Input: dimensioned drawing with shaded views. Units: mm. Origin: part minimum x, y, z. Round coordinates to 2 decimals unless told otherwise and drop trailing zeros. Answer as CSV lines item,"result". Start each with the question number.
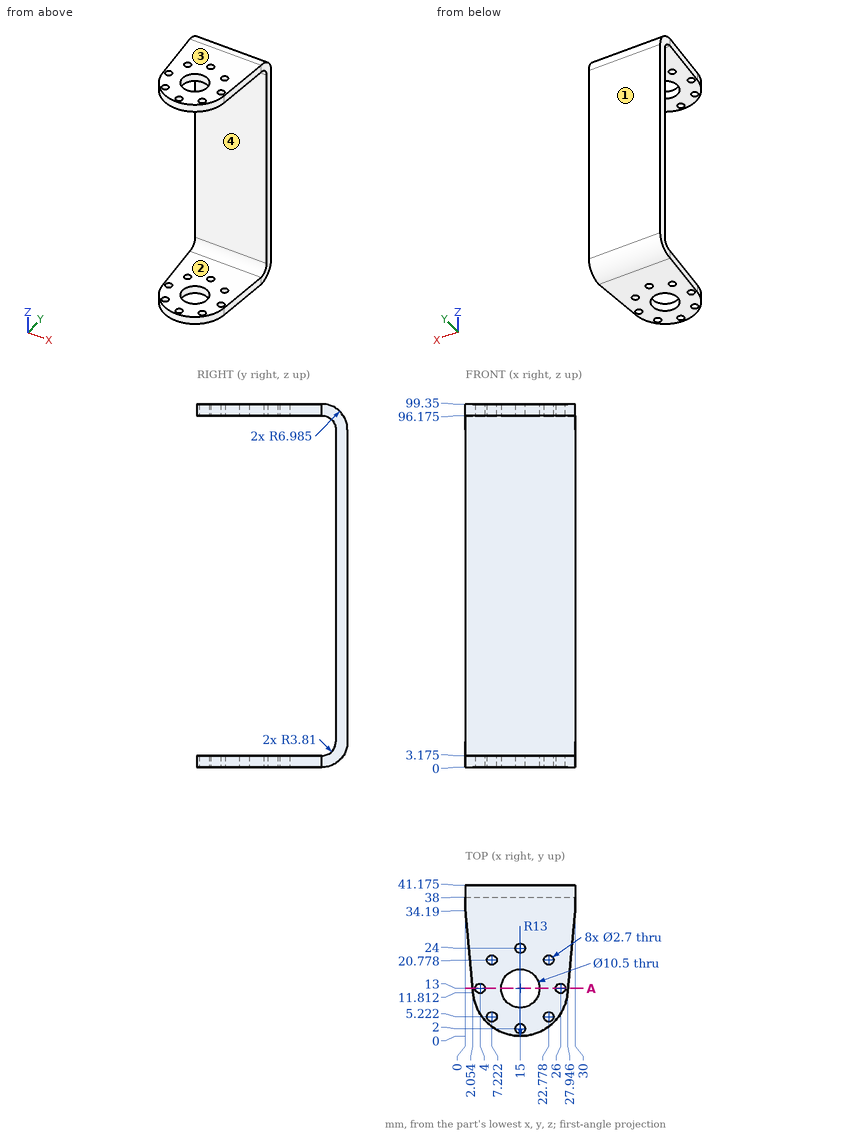
1) Section A-A, the plane y = 13. Give the number of separate pieces and of enclosed holes in the cut face.
2) Ray query, line 1 along Z through (x, y) = (4.25, 34.5); line 2 along Y through (x, z) = (25.5, 50) (1 decimal); line 3 along Z through (x, y) = (15.75, 37) (1 decimal). Return the intervals inside material, ascending.
3) Mould query, pull axis Z, two halves, no side actions, for the marked faces 1, 2, 3 and 4. Classes: pulls with the +Z half, pulls with the -Z half, needs draft (parallel to the pull), parting line crosses it, or undercut.
4) Contact query for a flat-ended pin moving along its axis: pin 1 Ø1 at (x, z) = (4.5, 47) entering from -Y. Output: stop coordinate, or through.
Findings below:
1,separate pieces,"8"
1,enclosed holes,"0"
2,line 1,"0.01 to 3.19, 96.16 to 99.34"
2,line 2,"38 to 41.2"
2,line 3,"0.6 to 4.4, 94.9 to 98.8"
3,face 1,"needs draft"
3,face 2,"undercut"
3,face 3,"pulls with the +Z half"
3,face 4,"undercut"
4,pin 1,"y = 38"
